Part print with two shaded views. Sizes in mm from the minimum x, y, z corner. Coordinates: 2 decimals unless noted, no trailing zeros. Loops run counter-clockwise (first coordinate to the right, second up) from the corner with the lowest first, then second, coordinate; pieces in that order, holes last. Notation, with made-up numbers: M -21.75,-25.75 L 25.25,-25.75 A15 ccw 25.25,-18.75 Z; hole C 53,81.25 d6. An arc over 180 degrees is marked long. Use CSV: the item, a comma, the result in double quotes. Start each with the question number.
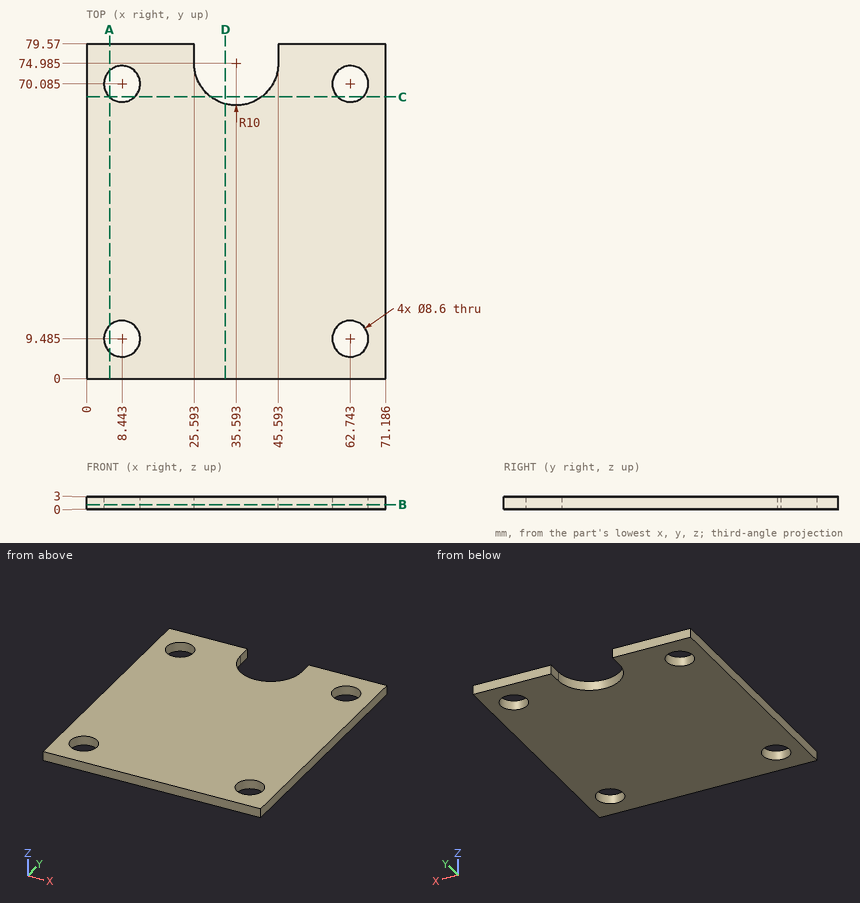
1. Slice it at C-C, the plane y = 67. List the corners of the cut face in (x, z) (1 decimal).
2. Slice it at D-D, the plane x = 33. List the corners of the cut face in (y, z), and give its area (3 significant figures).
3. Wall check: probe 1 along X at (y, z) = (66.5, 1.3) (1 decimal); probe 2 along X at (y, z) = (11, 1.35) (1 decimal); probe 3 along X at (y, z) = (68.5, 0.2) (1 decimal). Give the ranges that are in metal, low to high.
4. Slice it at B-B, the plane z = 1.1. List the corners of the cut face in (x, y) (1 decimal), and give its area (3 significant figures).
5. Slice it at A-A, the plane x = 5.5. List the corners of the cut face in (y, z).
Found:
1,outline,"M 0,0 L 5.4,0 L 5.4,3 L 0,3 Z; M 11.4,0 L 29.6,0 L 29.6,3 L 11.4,3 Z; M 41.6,0 L 59.7,0 L 59.7,3 L 41.6,3 Z; M 65.7,0 L 71.2,0 L 71.2,3 L 65.7,3 Z"
2,outline,"M 0,0 L 65.33,0 L 65.33,3 L 0,3 Z"
2,area,"196 mm^2"
3,probe 1,"0 to 6.1, 10.8 to 30.3, 40.9 to 60.4, 65.1 to 71.2"
3,probe 2,"0 to 4.4, 12.5 to 58.7, 66.8 to 71.2"
3,probe 3,"0 to 4.4, 12.4 to 28, 43.2 to 58.7, 66.7 to 71.2"
4,outline,"M 0,0 L 71.2,0 L 71.2,79.6 L 45.6,79.6 L 45.6,75 A10 cw 25.6,75 L 25.6,79.6 L 0,79.6 Z; hole C 8.4,9.5 d8.6; hole C 8.4,70.1 d8.6; hole C 62.7,9.5 d8.6; hole C 62.7,70.1 d8.6"
4,area,"5,180 mm^2"
5,outline,"M 0,0 L 6.35,0 L 6.35,3 L 0,3 Z; M 12.62,0 L 66.95,0 L 66.95,3 L 12.62,3 Z; M 73.22,0 L 79.57,0 L 79.57,3 L 73.22,3 Z"
